The model under review builds one solid part; all positions refer to its coordinate system, in mm. Coordinates: 2 decimals unless noted, no trailing zeros. Order: outer loops, then holes, each group sorted by start corner. A loop starts at its lowest first (then second) coordinate and runs counter-clockwise, first axis right, second up. Notation, with made-up numbers: (5, 20.25) -> (11, 20.25) arc R32 ccw to (11, 52.25) -> close; hole circle Ø9 at (15.25, 86). An arc over 180 degrees is marked (long way). Use one line per item in the form item = value. Start each with the question number.
(1) Take a section at A-A (x = -139). State the section outline as (y, z) points (3 decimals), then the cut area to 3 significant figures.
(2) Insertion check: pin 1 Ø1.6 at (x, y) = (-185.5, 1.5) entering from -Z. The pin has a flat end and moves straight along its axis. Give the tip position at first contact, or say it passes through.
(3) Take a section at C-C (x = -62). State the section outline as (y, z) points (3 decimals), then the cut area to 4 significant figures.
(4) Take a section at B-B (z = -65.5). State the section outline as (x, y) points (3 decimals).
(5) Wall thickness on line 1 along X through (y, z) = (2.8, -62); line 2 along Z through (x, y) = (-148, 0.85); line 3 along Z through (x, y) = (228.5, 1.3): over which ranges is each line inside the solid? List them lowest first.
(6) Take a section at D-D (y = 0.6). State how many separate pieces and enclosed holes the cut face has, then the cut area to 3 significant figures.
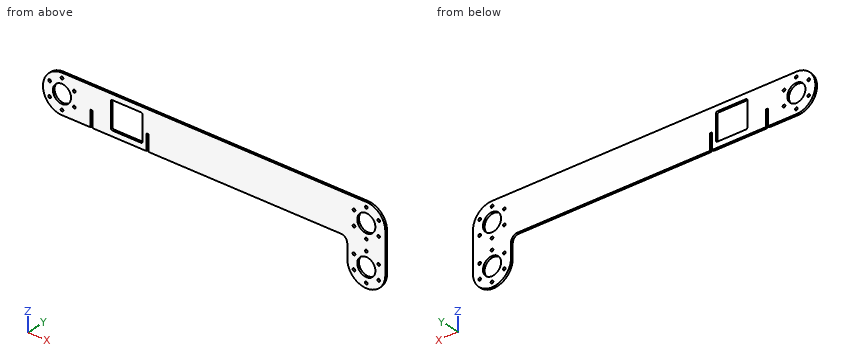
```python
from build123d import *

# Parameters (mm, degrees)
BOSS_EXTRUDE1_DEPTH = 3.175
SKETCH2_R           = 14.3
CUT_EXTRUDE1_DEPTH  = 293.296998547
SKETCH4_R           = 2.1
CUT_EXTRUDE2_DEPTH  = 293.296998547
SKETCH6_W           = 3.175
SKETCH6_H           = 25
CUT_EXTRUDE3_DEPTH  = 10
CUT_EXTRUDE6_DEPTH  = 10
SKETCH10_W          = 3.175
SKETCH10_H          = 25
CUT_EXTRUDE7_DEPTH  = 6.35


with BuildPart() as part:
    # Sketch1 → Boss-Extrude1 (new body)
    with BuildSketch(Plane(origin=(0, 0, 0), x_dir=(1, 0, 0), z_dir=(0, 1, 0))):
        with BuildLine():
            Line((277.741935484, -0.967741935), (277.741935484, 61.032258065))
            ThreePointArc((277.741935484, 61.032258065), (247.741935484, 91.032258065), (217.741935484, 61.032258065))
            Line((217.741935484, 61.032258065), (217.741935484, 39.032258065))
            ThreePointArc((217.741935484, 39.032258065), (214.813003296, 31.961190253), (207.741935484, 29.032258065))
            Line((207.741935484, 29.032258065), (-232.258064516, 29.032258065))
            ThreePointArc((-232.258064516, 29.032258065), (-262.258064516, -0.967741935), (-232.258064516, -30.967741935))
            Line((-232.258064516, -30.967741935), (247.741935484, -30.967741935))
            ThreePointArc((247.741935484, -30.967741935), (268.955138919, -22.180945371), (277.741935484, -0.967741935))
        make_face()
    extrude(amount=BOSS_EXTRUDE1_DEPTH)

    # Sketch2 → Cut-Extrude1 (cut, through all)
    with BuildSketch(Plane(origin=(0, 3.175, 0), x_dir=(1, 0, 0), z_dir=(0, 1, 0))):
        with Locations(Location((-232.258064516, -0.967741935, 0), (0, 0, 270))):
            Circle(SKETCH2_R)
        with Locations(Location((247.741935484, -0.967741935, 0), (0, 0, 270))):
            Circle(SKETCH2_R)
        with Locations(Location((247.741935484, 61.032258065, 0), (0, 0, 270))):
            Circle(SKETCH2_R)
    extrude(amount=-CUT_EXTRUDE1_DEPTH, mode=Mode.SUBTRACT)

    # Sketch4 → Cut-Extrude2 (cut, through all)
    with BuildSketch(Plane(origin=(0, 3.175, 0), x_dir=(1, 0, 0), z_dir=(0, 1, 0))):
        with Locations(Location((-232.258064516, 21.532258065, 0), (0, 0, 270))):
            Circle(SKETCH4_R)
        with Locations(Location((-212.772492931, 10.282258065, 0), (0, 0, 270))):
            Circle(SKETCH4_R)
        with Locations(Location((-212.772492931, -12.217741935, 0), (0, 0, 270))):
            Circle(SKETCH4_R)
        with Locations(Location((-232.258064516, -23.467741935, 0), (0, 0, 270))):
            Circle(SKETCH4_R)
        with Locations(Location((247.741935484, 83.532258065, 0), (0, 0, 270))):
            Circle(SKETCH4_R)
        with Locations(Location((247.741935484, 21.532258065, 0), (0, 0, 270))):
            Circle(SKETCH4_R)
        with Locations(Location((267.227507069, 72.282258065, 0), (0, 0, 270))):
            Circle(SKETCH4_R)
        with Locations(Location((267.227507069, 49.782258065, 0), (0, 0, 270))):
            Circle(SKETCH4_R)
        with Locations(Location((247.741935484, 38.532258065, 0), (0, 0, 270))):
            Circle(SKETCH4_R)
        with Locations(Location((267.227507069, 10.282258065, 0), (0, 0, 270))):
            Circle(SKETCH4_R)
        with Locations(Location((267.227507069, -12.217741935, 0), (0, 0, 270))):
            Circle(SKETCH4_R)
        with Locations(Location((247.741935484, -23.467741935, 0), (0, 0, 270))):
            Circle(SKETCH4_R)
        with Locations(Location((-251.743636101, -12.217741935, 0), (0, 0, 270))):
            Circle(SKETCH4_R)
        with Locations(Location((-251.743636101, 10.282258065, 0), (0, 0, 270))):
            Circle(SKETCH4_R)
        with Locations(Location((228.256363899, -12.217741935, 0), (0, 0, 270))):
            Circle(SKETCH4_R)
        with Locations(Location((228.256363899, 10.282258065, 0), (0, 0, 270))):
            Circle(SKETCH4_R)
        with Locations(Location((228.256363899, 49.782258065, 0), (0, 0, 270))):
            Circle(SKETCH4_R)
        with Locations(Location((228.256363899, 72.282258065, 0), (0, 0, 270))):
            Circle(SKETCH4_R)
    extrude(amount=-CUT_EXTRUDE2_DEPTH, mode=Mode.SUBTRACT)

    # Sketch6 → Cut-Extrude3 (cut)
    with BuildSketch(Plane(origin=(0, 3.175, 0), x_dir=(1, 0, 0), z_dir=(0, 1, 0))):
        with Locations((-185.670564516, 16.532258065)):
            Rectangle(SKETCH6_W, SKETCH6_H)
    extrude(amount=-CUT_EXTRUDE3_DEPTH, mode=Mode.SUBTRACT)

    # Sketch9 → Cut-Extrude6 (cut)
    with BuildSketch(Plane(origin=(0, 3.175, 0), x_dir=(1, 0, 0), z_dir=(0, 1, 0))):
        with BuildLine():
            Line((-148.258064516, -22.467741935), (-107.689679667, -22.467741935))
            ThreePointArc((-107.689679667, -22.467741935), (-105.970268104, -21.755538347), (-105.258064516, -20.036126785))
            Line((-105.258064516, -20.036126785), (-105.258064516, 18.100642914))
            ThreePointArc((-105.258064516, 18.100642914), (-105.970268104, 19.820054476), (-107.689679667, 20.532258065))
            Line((-107.689679667, 20.532258065), (-148.258064516, 20.532258065))
            Line((-148.258064516, 20.532258065), (-152.826449366, 20.532258065))
            ThreePointArc((-152.826449366, 20.532258065), (-154.545860928, 19.820054476), (-155.258064516, 18.100642914))
            Line((-155.258064516, 18.100642914), (-155.258064516, -20.036126785))
            ThreePointArc((-155.258064516, -20.036126785), (-154.545860928, -21.755538347), (-152.826449366, -22.467741935))
            Line((-152.826449366, -22.467741935), (-148.258064516, -22.467741935))
        make_face()
    extrude(amount=-CUT_EXTRUDE6_DEPTH, mode=Mode.SUBTRACT)

    # Sketch10 → Cut-Extrude7 (cut)
    with BuildSketch(Plane(origin=(0, 3.175, 0), x_dir=(1, 0, 0), z_dir=(0, 1, 0))):
        with Locations((-97.670564516, 16.532258065)):
            Rectangle(SKETCH10_W, SKETCH10_H)
    extrude(amount=-CUT_EXTRUDE7_DEPTH, mode=Mode.SUBTRACT)


solid = part.part
```
Findings:
q1.outline = (0, -29.032) -> (3.175, -29.032) -> (3.175, -20.532) -> (0, -20.532) -> close; (0, 22.468) -> (3.175, 22.468) -> (3.175, 30.968) -> (0, 30.968) -> close
q1.area = 54.0 mm²
q2.pin_1 = -4.03
q3.outline = (0, -29.032) -> (3.175, -29.032) -> (3.175, 30.968) -> (0, 30.968) -> close
q3.area = 190.5 mm²
q4.outline = (218.076, 0) -> (234.158, 0) -> (234.158, 3.175) -> (218.076, 3.175) -> close; (261.326, 0) -> (277.407, 0) -> (277.407, 3.175) -> (261.326, 3.175) -> close
q5.line_1 = 217.76 to 233.47, 262.01 to 277.73
q5.line_2 = -29.03 to -20.53, 22.47 to 30.97
q5.line_3 = -84.05 to -74.37, -70.2 to -51.87, -47.7 to -12.37, -8.2 to 10.13, 14.3 to 30.97
q6.separate_pieces = 1
q6.enclosed_holes = 22
q6.area = 30,700 mm²
